Could you check a few things on this model? Use its own coordinates, in mm. A direction names the side the tool comes from. Coordinates: 2 decimals unless noted, no trailing zeros. Loops run counter-clockwise (first coordinate to the right, second up) from the corner with the lowest first, then second, coordinate; pieces in that order, holes last. Notation, with made-up numbers: (-5.75, -23.5) -> (10.25, -23.5) arc R22 ccw to (10.25, 1.5) -> close; hole circle Ø6 at (7.25, -36). An arc over 180 degrees is marked (long way). One line per question, with ' | ' between items.
from build123d import *

# Parameters (mm, degrees)
BOSS_EXTRUDE1_DEPTH      = 2
BOSS_EXTRUDE1_DEPTH_BACK = 4
SKETCH1_W                = 12.8
SKETCH1_H                = 15.5
SKETCH2_W                = 15.5
SKETCH2_H                = 4
SKETCH2_H_2              = 22.7
SKETCH2_H_3              = 2
BOSS_EXTRUDE2_DEPTH      = 2.5
BOSS_EXTRUDE3_DEPTH      = 2.5
SKETCH5_W                = 17.8
SKETCH5_H                = 60.5
BOSS_EXTRUDE5_DEPTH      = 2.5


with BuildPart() as part:
    # Sketch1 → Boss-Extrude1 (new, two sides: drawn at the far end of the back side and taken through both)
    with BuildSketch(Plane(origin=(0, 0, 0), x_dir=(1, 0, 0), z_dir=(0, 1, 0)).offset(-BOSS_EXTRUDE1_DEPTH_BACK)):
        with Locations((6.4, 7.75)):
            Rectangle(SKETCH1_W, SKETCH1_H)
    extrude(amount=BOSS_EXTRUDE1_DEPTH + BOSS_EXTRUDE1_DEPTH_BACK)

    # Sketch2 → Boss-Extrude2 (add)
    with BuildSketch(Plane(origin=(12.8, 0, 0), x_dir=(0, 0, -1), z_dir=(1, 0, 0))):
        with Locations((7.75, -2)):
            Rectangle(SKETCH2_W, SKETCH2_H)
        with Locations((7.75, 13.35)):
            Rectangle(SKETCH2_W, SKETCH2_H_2)
        with Locations((7.75, 1)):
            Rectangle(SKETCH2_W, SKETCH2_H_3)
    extrude(amount=BOSS_EXTRUDE2_DEPTH)

    # Sketch3 → Boss-Extrude3 (add)
    with BuildSketch(Plane.ZY):
        Polygon((0, 0), (0, 24.7), (-15.5, 24.7), (-15.5, 0), (-15.5, -4), (0, -4), align=None)
    extrude(amount=BOSS_EXTRUDE3_DEPTH)

    # Sketch5 → Boss-Extrude5 (add)
    with BuildSketch(Plane.XZ.offset(4)):
        with Locations((6.4, 14.75)):
            Rectangle(SKETCH5_W, SKETCH5_H)
    extrude(amount=BOSS_EXTRUDE5_DEPTH)


solid = part.part
1) On a 3-axis mill with a long thin cutter (end or side, diameter ignored), from which of +Z, -Z, +X, -X, +Y, -Y can I reach the whole of each face in a straight line? I mean faces 1 (the face through (6, 2, -8)), 2 (the face through (6, -5, 45)), 3 (the face through (6, -4, 23)). Say none if no direction works.
Data:
face 1: +Z, -Z, +Y | face 2: +Z, +X, -X, +Y, -Y | face 3: +Z, +X, -X, +Y
2) If we section it at B-B on z = -6: Please give me the cut outline in (x, y).
Data:
outline: (-2.5, -6.5) -> (15.3, -6.5) -> (15.3, 24.7) -> (12.8, 24.7) -> (12.8, 2) -> (0, 2) -> (0, 24.7) -> (-2.5, 24.7) -> close
3) If we section it at D-D on y = -1.5: Please give me the cut outline in (x, z).
Data:
outline: (-2.5, -15.5) -> (15.3, -15.5) -> (15.3, 0) -> (-2.5, 0) -> close
4) If we section it at C-C on x = 3.75: Please give me the cut outline in (y, z).
Data:
outline: (-6.5, -15.5) -> (2, -15.5) -> (2, 0) -> (-4, 0) -> (-4, 45) -> (-6.5, 45) -> close
5) I need wall thicknesses on line 1 along X through (y, z) = (23.5, -5); line 2 along Y through (x, z) = (4.25, 9.5); line 3 along Z through (x, y) = (14.25, 14). Which ranges of each line are inside material? Lowest first, please. Write a range as from..to.
Data:
line 1: -2.5..0, 12.8..15.3 | line 2: -6.5..-4 | line 3: -15.5..0
6) I'm going to push flat-ended pins straight in: pin 1 Ø1 at (x, z) = (9, 25) entering from +Y; pin 2 Ø6.5 at (x, z) = (8, -8.5) entering from +Y. Where does each tip first touch, or does it pass through?
Data:
pin 1: y = -4 | pin 2: y = 2
7) If we section it at A-A on y = 6: Please give me the cut outline in (x, z), and give its area (3 significant figures).
Data:
outline: (-2.5, -15.5) -> (0, -15.5) -> (0, 0) -> (-2.5, 0) -> close; (12.8, -15.5) -> (15.3, -15.5) -> (15.3, 0) -> (12.8, 0) -> close | area: 77.5 mm²
